from build123d import *

# Parameters (mm, degrees)
PLAT_W                      = 30
PLAT_H                      = 15
EL_MENT_M_CANO_SOUD_1_DEPTH = 470
ENL_V_MAT_EXTRU_2_DEPTH     = 20
R_P_TITION_LIN_AIRE1_COUNT  = 4
R_P_TITION_LIN_AIRE1_PITCH  = 140


with BuildPart() as part:
    # plat → Elément mécano-soudé1 (new body)
    with BuildSketch(Plane.YZ.offset(-235)):
        Rectangle(PLAT_W, PLAT_H)
    extrude(amount=EL_MENT_M_CANO_SOUD_1_DEPTH)

    # Esquisse7 → Enlèv. mat.-Extru.2 (cut)
    with BuildSketch(Plane.XY.offset(7.5)):
        with BuildLine():
            Line((-215.5, -5), (-215.5, 5))
            ThreePointArc((-215.5, 5), (-210, 10.5), (-204.5, 5))
            Line((-204.5, 5), (-204.5, -5))
            ThreePointArc((-204.5, -5), (-210, -10.5), (-215.5, -5))
        make_face()
    enl_v_mat_extru_2 = extrude(amount=-ENL_V_MAT_EXTRU_2_DEPTH, mode=Mode.SUBTRACT)

    # Répétition linéaire1: Enlèv. mat.-Extru.2 ×4
    with Locations(*[(i * R_P_TITION_LIN_AIRE1_PITCH, 0, 0) for i in range(1, R_P_TITION_LIN_AIRE1_COUNT)]):
        add(enl_v_mat_extru_2, mode=Mode.SUBTRACT)


solid = part.part
Verification items for the finished model (mm, model axes). A direction names the side the tool comes from. Coordinates: 2 decimals unless noted, no trailing zeros. Order: outer loops, then holes, each group sorted by start corner. A loop starts at its lowest first (then second) coordinate and runs counter-clockwise, first axis right, second up. Notation, with made-up numbers: M -32,-25 L -23,-25 A24 cw -23,-2 Z; hole C 78,21 d8. An arc over 180 degrees is marked long. Return JSON: item names as keys, results as strings.
1) Release check for a two-part mould opening along Y. For faces 3 (the flat face through (215.5, 0, 0)), 4 (the cylindrical face through (69.9, 10.5, 0.1)), 5 (the flat face through (-3, -15, 0)), 6 (the flat face through (-235, 0, 0)) record: +Y half, -Y half, draft (parallel to the pull), parting line (faces both ways), or undercut.
Answer list:
{"face 3": "undercut", "face 4": "undercut", "face 5": "-Y half", "face 6": "draft"}
2) Access from +Z, -Z, +X, -X, +Y, -Y to the whole of each face (thin tool, end or side, straight path). Record for faces 1 (the flat face through (235, 0, 0)), 2 (the flat face through (-204.5, 0, 0)).
Answer list:
{"face 1": "+Z, -Z, +X, +Y, -Y", "face 2": "+Z, -Z"}
3) Thickness scan on L1, parallel to X at y = -6, z = -5.25; L2, parallel to X at y = -3.5, z = -1.5; L3, parallel to Y at x = 210, z = 6.5. Record the ranges inside material, lowest first. Write a range as [from, to].
Answer list:
{"L1": "[-235, -215.41], [-204.59, -75.41], [-64.59, 64.59], [75.41, 204.59], [215.41, 235]", "L2": "[-235, -215.5], [-204.5, -75.5], [-64.5, 64.5], [75.5, 204.5], [215.5, 235]", "L3": "[-15, -10.5], [10.5, 15]"}
4) Cross-section at B-B, the plane x = 210. Record the boundary of the cut face in (y, z), and give its area (3 significant figures).
Answer list:
{"outline": "M -15,-7.5 L -10.5,-7.5 L -10.5,7.5 L -15,7.5 Z; M 10.5,-7.5 L 15,-7.5 L 15,7.5 L 10.5,7.5 Z", "area": "135 mm2"}
5) Cross-section at A-A, the plane y = 1. Record the boundary of the cut face in (x, z), and give its area (3 significant figures).
Answer list:
{"outline": "M -235,-7.5 L -215.5,-7.5 L -215.5,7.5 L -235,7.5 Z; M -204.5,-7.5 L -75.5,-7.5 L -75.5,7.5 L -204.5,7.5 Z; M -64.5,-7.5 L 64.5,-7.5 L 64.5,7.5 L -64.5,7.5 Z; M 75.5,-7.5 L 204.5,-7.5 L 204.5,7.5 L 75.5,7.5 Z; M 215.5,-7.5 L 235,-7.5 L 235,7.5 L 215.5,7.5 Z", "area": "6,390 mm2"}
6) Cross-section at C-C, the plane z = 3.75. Record the boundary of the cut face in (x, y), and give its area (3 significant figures).
Answer list:
{"outline": "M -235,-15 L 235,-15 L 235,15 L -235,15 Z; hole M -215.5,-5 A5.5 ccw -204.5,-5 L -204.5,5 A5.5 ccw -215.5,5 Z; hole M -75.5,-5 A5.5 ccw -64.5,-5 L -64.5,5 A5.5 ccw -75.5,5 Z; hole M 64.5,-5 A5.5 ccw 75.5,-5 L 75.5,5 A5.5 ccw 64.5,5 Z; hole M 204.5,-5 A5.5 ccw 215.5,-5 L 215.5,5 A5.5 ccw 204.5,5 Z", "area": "13,300 mm2"}
